Drawing for the job (mm, zero at the part's lowest x, y, z). Give positions to 0.01 mm unless a question says otherwise; leave off trailing zeros. Loops run counter-clockwise (first coordinate to the right, second up) from the corner with the lowest first, then second, coordinate; pieces in that order, holes last.
1) Flat gauge pins, fed straight in: P1, Ø1.5, axis at x = 8, z = 4.5, coming from the -Y side; P2, Ø3, axis at x = 8, z = 4.5, coming from the -Y side; P3, Ø8, axis at x = 19.5, z = 2.5, coming from the -Y side. Where does each tip first touch, or does it go through?
2) Wall check: line 1 (Y direction, x = 15.75, z = 7); line 2 (X direction, y = 5.5, z = 13); line 3 (Z direction, x = 2, y = 11.5). Give the ranges that are in metal, low to high.
3) Band-saw the part on C-C on x = 17.75. List the corners of the cut face in (y, z), then the cut area to 3 significant figures.
4) Band-saw the part on A-A on z = 7. List the corners of the cut face in (x, y), then the cut area to 3 significant figures.
5) Two-plate mould, pull along Z, no slides. Class the marked faces 1 and 2: +Z half, -Z half, draft (parallel to the pull), parting line (faces both ways), or undercut.
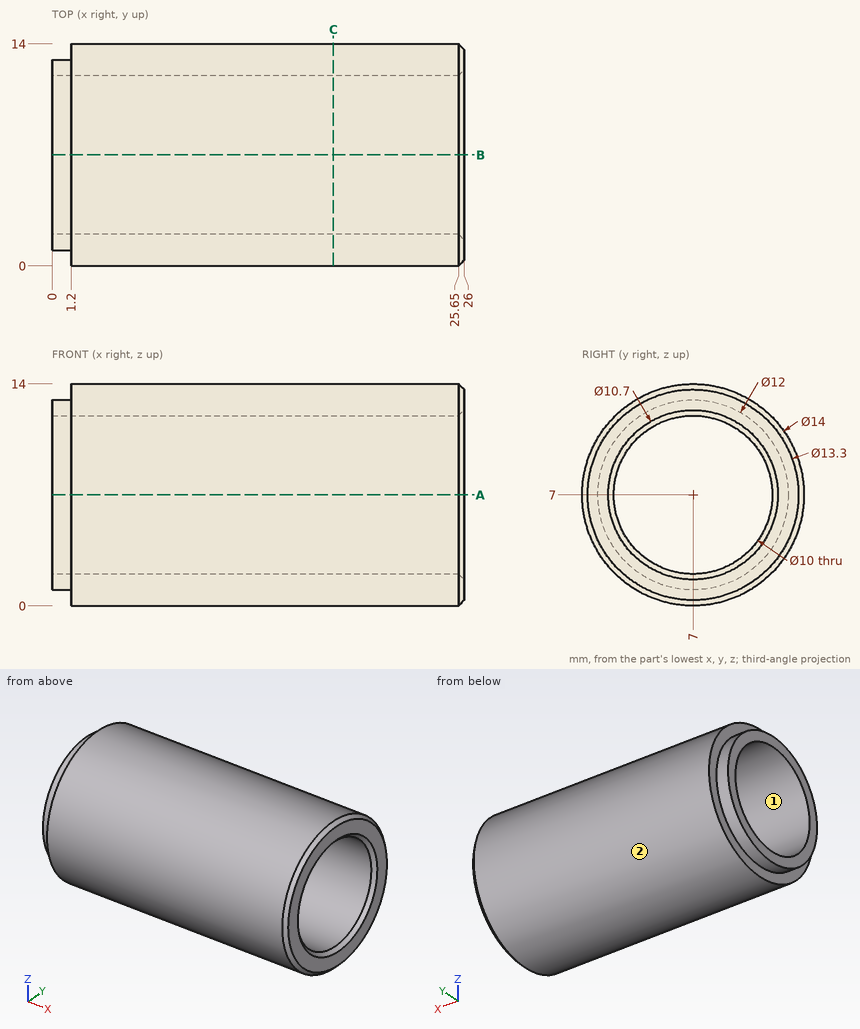
Findings below:
1. P1: stops at y = 0.22
1. P2: stops at y = 0.07
1. P3: stops at y = 0.02
2. line 1: y = 0 to 2, 12 to 14
2. line 2: x = 1.2 to 26
2. line 3: z = 1.64 to 4.82, 9.18 to 12.36
3. outline: circle Ø14 at (7, 7); hole circle Ø10 at (7, 7)
3. area: 75.4 mm2
4. outline: (0, 1) - (1.2, 1) - (1.2, 0) - (25.65, 0) - (26, 0.35) - (26, 1.65) - (25.65, 2) - (0, 2) - close; (0, 12) - (25.65, 12) - (26, 12.35) - (26, 13.65) - (25.65, 14) - (1.2, 14) - (1.2, 13) - (0, 13) - close
4. area: 101 mm2
5. face 1: undercut
5. face 2: parting line
